Work out the finished part from the listing and answer in its coordinate system (mm). Round coordinates to 2 decimals unless told otherwise and drop trailing zeros. Write each loop counter-clockwise with the first axis right and the second up, starting at its lowest first coordinate (ties: lowest second). Pieces come first, ordered by that corner, then holes.
from build123d import *

# Parameters (mm, degrees)
SKETCH_1_W      = 34
SKETCH_1_H      = 45.83
EXTRUDE_1_DEPTH = 2.25
SKETCH_2_W      = 28.03
SKETCH_2_H      = 35.04
EXTRUDE_2_DEPTH = 0.1
SKETCH_4_W      = 0.4
SKETCH_4_H      = 1.8
EXTRUDE_3_DEPTH = 0.1


with BuildPart() as part:
    # Эскиз1 → Бобышка-Вытянуть1 (new body)
    with BuildSketch(Plane(origin=(0, 0, 0), x_dir=(1, 0, 0), z_dir=(0, 1, 0))):
        Rectangle(SKETCH_1_W, SKETCH_1_H)
    extrude(amount=EXTRUDE_1_DEPTH)

    # Эскиз2 → Бобышка-Вытянуть2 (add)
    with BuildSketch(Plane(origin=(0, 2.25, 0), x_dir=(1, 0, 0), z_dir=(0, 1, 0))):
        with Locations((0, 2.565)):
            Rectangle(SKETCH_2_W, SKETCH_2_H)
    extrude(amount=EXTRUDE_2_DEPTH)

    # Эскиз4 → Бобышка-Вытянуть3 (add)
    with BuildSketch(Plane.XZ):
        with Locations((-4.4, 13.564176084)):
            Rectangle(SKETCH_4_W, SKETCH_4_H)
        with Locations((-5.2, 13.564176084)):
            Rectangle(SKETCH_4_W, SKETCH_4_H)
        with Locations((-3.6, 13.564176084)):
            Rectangle(SKETCH_4_W, SKETCH_4_H)
        with Locations((-2.8, 13.564176084)):
            Rectangle(SKETCH_4_W, SKETCH_4_H)
        with Locations((-2, 13.564176084)):
            Rectangle(SKETCH_4_W, SKETCH_4_H)
        with Locations((-1.2, 13.564176084)):
            Rectangle(SKETCH_4_W, SKETCH_4_H)
        with Locations((-0.4, 13.564176084)):
            Rectangle(SKETCH_4_W, SKETCH_4_H)
        with Locations((0.4, 13.564176084)):
            Rectangle(SKETCH_4_W, SKETCH_4_H)
        with Locations((1.2, 13.564176084)):
            Rectangle(SKETCH_4_W, SKETCH_4_H)
        with Locations((2, 13.564176084)):
            Rectangle(SKETCH_4_W, SKETCH_4_H)
        with Locations((2.8, 13.564176084)):
            Rectangle(SKETCH_4_W, SKETCH_4_H)
        with Locations((3.6, 13.564176084)):
            Rectangle(SKETCH_4_W, SKETCH_4_H)
        with Locations((4.4, 13.564176084)):
            Rectangle(SKETCH_4_W, SKETCH_4_H)
        with Locations((5.2, 13.564176084)):
            Rectangle(SKETCH_4_W, SKETCH_4_H)
    extrude(amount=EXTRUDE_3_DEPTH)


solid = part.part
Q1. Find the intervals of material crossed by L1, parallel to Y at x = -3.5, z = -8.5; L2, parallel to Y at x = 12.5, z = 18, in increasing order.
Q2. Find section A-A (z = 6). Determine the outline of the cut face in (x, y) (3 decimals).
Q3. Find section B-B (x = 11.5). Determine the outline of the cut face in (y, z) (3 decimals).
Q4. Given pin 1 (2 mm diameter, centred on x = 6.5, z = -17.5, fed in from -Y), flat-ended and moving along its own axis, determine where the tip first touches the part or whether it passes through.
Report:
1. L1: y = 0 to 2.35
1. L2: y = 0 to 2.25
2. outline: (-17, 0) - (17, 0) - (17, 2.25) - (14.015, 2.25) - (14.015, 2.35) - (-14.015, 2.35) - (-14.015, 2.25) - (-17, 2.25) - close
3. outline: (0, -22.915) - (2.25, -22.915) - (2.25, -20.085) - (2.35, -20.085) - (2.35, 14.955) - (2.25, 14.955) - (2.25, 22.915) - (0, 22.915) - close
4. pin 1: stops at y = 0
